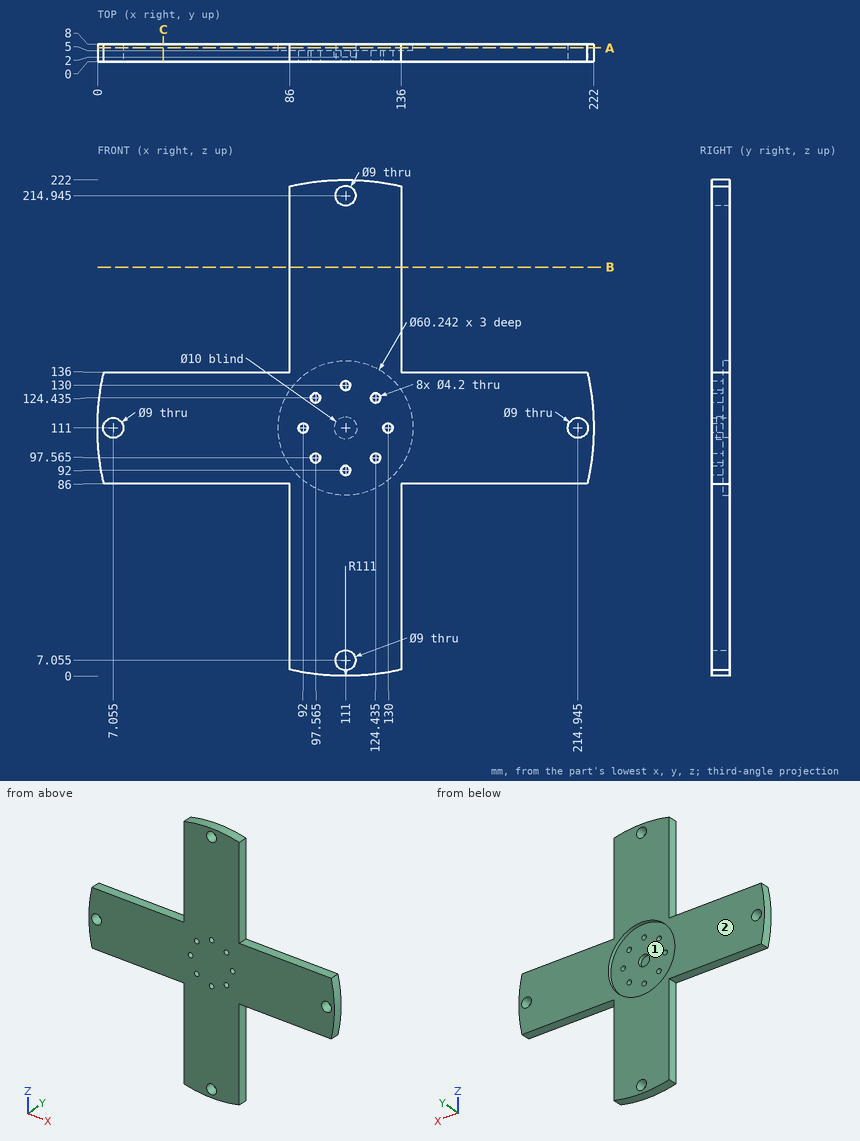
Answer from the drawing. Dimensions are ordinates in mm from the lowest x, y and z of the part. Coordinates: 2 decimals unless noted, no trailing zeros. Order: outer loops, then holes, each group sorted by start corner. A loop starts at its lowest first (then second) coordinate and runs counter-clockwise, first axis right, second up. Notation, with made-up numbers: (81.25, 71) - (90.25, 71) arc R33 cw to (90.25, 103) - close; hole circle Ø10 at (26, 14.5). An arc over 180 degrees is marked (long way). Use one line per item in the form item = value.
(1) Section A-A, the plane y = 6.25 is taken. Give the vertices of the cut face in (x, z) (1 decimal), then the cut area to 3 significant figures.
Computed values:
outline = (2.9, 86) - (86, 86) - (86, 2.9) arc R111 ccw to (136, 2.9) - (136, 86) - (219.1, 86) arc R111 ccw to (219.1, 136) - (136, 136) - (136, 219.1) arc R111 ccw to (86, 219.1) - (86, 136) - (2.9, 136) arc R111 ccw to start; hole circle Ø9 at (7.1, 111); hole circle Ø60.2 at (111, 111); hole circle Ø9 at (111, 7.1); hole circle Ø9 at (111, 214.9); hole circle Ø9 at (214.9, 111)
area = 16,400 mm²
(2) Section B-B, the plane z = 183 is taken. Give the vertices of the cut face in (x, y), then the cut area to 3 significant figures.
Computed values:
outline = (86, 0) - (136, 0) - (136, 8) - (86, 8) - close
area = 400 mm²
(3) Straight lines are drawn through the part: L1, parallel to Y at x = 106, z = 108; L2, parallel to Z at x = 165, y = 1.5. For each, find the intervals that lie inside material, in ascending order.
Computed values:
L1 = 0 to 5
L2 = 86 to 136
(4) Given pin 1 Ø1.5 at (y, z) = (6, 66.5) entering from -X; pin 2 Ø4 at (y, z) = (1.5, 95) entering from +X; pin 3 Ø4 at (x, y) = (130.5, 5.5) entering from +Z, each flat-ended and moving along its own axis, determine where each tip first touches the part or whether it passes through.
Computed values:
pin_1 = 86
pin_2 = 221.11
pin_3 = 220.61
(5) Section C-C, the plane x = 29.5 is taken. Give the vertices of the cut face in (y, z), then the cut area to 3 significant figures.
Computed values:
outline = (0, 86) - (8, 86) - (8, 136) - (0, 136) - close
area = 400 mm²
(6) For a pull along X with two mould halves and no side action, classify the marked faces 1 and 2 as pulls with the +X half, pulls with the -X half, needs draft (parallel to the pull), parting line crosses it, or undercut.
Computed values:
face_1 = undercut
face_2 = needs draft
